```python
from build123d import *

# Parameters (mm, degrees)
F0_R     = 1
F1_DEPTH = 1.5
F3_DEPTH = 1.5
F4_W     = 1.5
F4_H     = 24
F5_DEPTH = 14.65


with BuildPart() as f1:
    # F0 (on Top) → F1 (new body)
    with BuildSketch(Plane.XY):
        with BuildLine():
            Line((-4, 16), (-16.22254, 16))
            Line((-16.22254, 16), (-16.22254, -16))
            Line((-16.22254, -16), (-4, -16))
            Line((-4, -16), (-4, -13))
            ThreePointArc((-4, -13), (0, -9), (4, -13))
            Line((4, -13), (4, -16))
            Line((4, -16), (16.22254, -16))
            Line((16.22254, -16), (16.22254, 16))
            Line((16.22254, 16), (4, 16))
            Line((4, 16), (4, 13))
            ThreePointArc((4, 13), (0, 9), (-4, 13))
            Line((-4, 13), (-4, 16))
        make_face()
        with Locations((-6.22254, -13)):
            Circle(F0_R, mode=Mode.SUBTRACT)
        with Locations((-4.4, -8.6)):
            Circle(F0_R, mode=Mode.SUBTRACT)
        with Locations((6.22254, -13)):
            Circle(F0_R, mode=Mode.SUBTRACT)
        with Locations((4.4, -8.6)):
            Circle(F0_R, mode=Mode.SUBTRACT)
        with Locations((0, -6.77746)):
            Circle(F0_R, mode=Mode.SUBTRACT)
        with Locations((-4.4, 8.6)):
            Circle(F0_R, mode=Mode.SUBTRACT)
        with Locations((-6.22254, 13)):
            Circle(F0_R, mode=Mode.SUBTRACT)
        with Locations((0, 6.77746)):
            Circle(F0_R, mode=Mode.SUBTRACT)
        with Locations((4.4, 8.6)):
            Circle(F0_R, mode=Mode.SUBTRACT)
        with Locations((6.22254, 13)):
            Circle(F0_R, mode=Mode.SUBTRACT)
    extrude(amount=F1_DEPTH)

    # F2 (on face) → F3 (cut, through all)
    with BuildSketch(Plane.XY.offset(1.5)):
        Polygon((16.22254, 16), (8.22254, 16), (16.22254, 4), align=None)
        Polygon((8.22254, -16), (16.22254, -16), (16.22254, -4), align=None)
        Polygon((-12.22254, 16), (-16.22254, 16), (-16.22254, 12), align=None)
        Polygon((-16.22254, -16), (-12.22254, -16), (-16.22254, -12), align=None)
    extrude(amount=-F3_DEPTH, mode=Mode.SUBTRACT)

    # F4 (on face) → F5 (join)
    with BuildSketch(Plane(origin=(0, 0, 0), x_dir=(1, 0, 0), z_dir=(0, 0, -1))):
        with Locations((-15.47254, 0)):
            Rectangle(F4_W, F4_H)
    extrude(amount=F5_DEPTH)

    # F7: F1 across plane


with BuildPart() as f1_1:
    add(f1.part)
    add(f1.part.mirror(Plane.XY.offset(-14.65)))


solid = f1_1.part
```
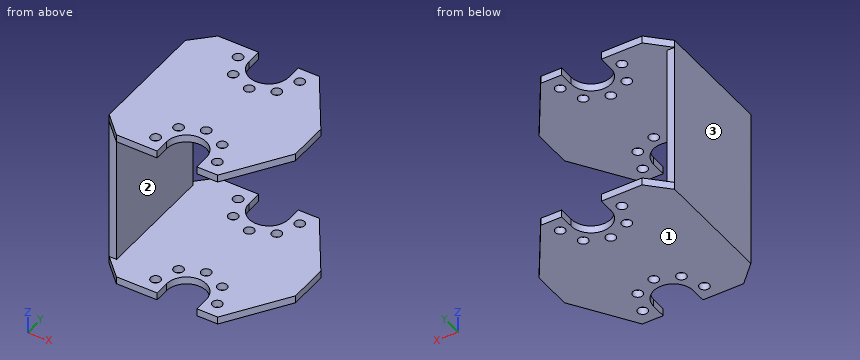
Source: CAD feature listing. Evaluate the final solid. Frame: model axes, mm. Face numbers are marked on the shaded views. Round coordinates to 2 decimals unless told otherwise and drop trailing zeros. Order: outer loops, then holes, each group sorted by start corner. A loop starts at its lowest first (then second) coordinate and runs counter-clockwise, first axis right, second up. Notation, with made-up numbers: (53, -30) -> (66, -30) arc R15 ccw to (66, -14) -> close; hole circle Ø7 at (-39.5, 57.25). An arc over 180 degrees is marked (long way). One line per item, written item: value. Start each with the question number.
Q1. Material intervals for probe 1 along Z at (x, y) = (11, -4); probe 2 along X at (y, z) = (8, -30); probe 3 along X at (y, z) = (-1.5, -11.5), sorted ascending.
Q2. Section query B-B (y = -0.5). Return the cut outline in (x, z).
Q3. Section query C-C (y = 11). Return the cut outline in (x, z), plus the area to 3 significant figures.
Q4. Section query A-A (x = 0). Return the cut outline in (y, z).
Q5. Draft query along Z for the marked faces 1, 2 and 3. Return one class per face: pulls with the +Z half, pulls with the -Z half, needs draft (parallel to the pull), parting line crosses it, or undercut.
Q6. Section query D-D (z = -11.5). Return the cut outline in (x, y), plus the area to 3 significant figures.
Q7. Pin query (flat end, axial travel): pin 1 (0.8 mm diameter, centred on y = 14, z = -30, fed in from +X); pin 2 (1.7 mm diameter, centred on x = -15.5, z = -15.5, fed in from -Y); pin 3 (12 mm diameter, centred on y = 9.5, z = -10.5, fed in from +X). Return the tip coordinate at first contact, or that it passes through.
Findings below:
1. probe 1: -30.8 to -29.3, 0 to 1.5
1. probe 2: -16.22 to -5.2, -3.6 to 3.6, 5.2 to 13.56
1. probe 3: -16.22 to -14.72
2. outline: (-16.22, -30.8) -> (16.22, -30.8) -> (16.22, -29.3) -> (-14.72, -29.3) -> (-14.72, 0) -> (16.22, 0) -> (16.22, 1.5) -> (-16.22, 1.5) -> close
3. outline: (-16.22, -30.8) -> (-3.46, -30.8) -> (-3.46, -29.3) -> (-14.72, -29.3) -> (-14.72, 0) -> (-3.46, 0) -> (-3.46, 1.5) -> (-16.22, 1.5) -> close; (3.46, -30.8) -> (11.56, -30.8) -> (11.56, -29.3) -> (3.46, -29.3) -> close; (3.46, 0) -> (11.56, 0) -> (11.56, 1.5) -> (3.46, 1.5) -> close
3. area: 107 mm²
4. outline: (-9, -30.8) -> (-7.78, -30.8) -> (-7.78, -29.3) -> (-9, -29.3) -> close; (-9, 0) -> (-7.78, 0) -> (-7.78, 1.5) -> (-9, 1.5) -> close; (-5.78, -30.8) -> (5.78, -30.8) -> (5.78, -29.3) -> (-5.78, -29.3) -> close; (-5.78, 0) -> (5.78, 0) -> (5.78, 1.5) -> (-5.78, 1.5) -> close; (7.78, -30.8) -> (9, -30.8) -> (9, -29.3) -> (7.78, -29.3) -> close; (7.78, 0) -> (9, 0) -> (9, 1.5) -> (7.78, 1.5) -> close
5. face 1: pulls with the -Z half
5. face 2: undercut
5. face 3: needs draft
6. outline: (-16.22, -12) -> (-14.72, -12) -> (-14.72, 12) -> (-16.22, 12) -> close
6. area: 36.0 mm²
7. pin 1: x = 9.82
7. pin 2: y = -12
7. pin 3: x = -14.72
